```python
from build123d import *

# Parameters (mm, degrees)
F3_START = 7.62
F2_R     = 4.826
F3_DEPTH = 93.981
F4_R     = 1.1938
F5_DEPTH = 12.7


with BuildPart() as f1:
    # F0 (on Right) → F1 (revolve)
    with BuildSketch(Plane.YZ):
        with BuildLine():
            Line((-40.64, 3.175), (0, 3.175))
            Line((0, 3.175), (0, 12.7))
            Line((0, 12.7), (-6.35, 12.7))
            Line((-6.35, 12.7), (-6.35, 9.7636567324))
            ThreePointArc((-6.35, 9.7636567324), (-7.4331158517, 7.6830105399), (-9.758731164, 7.3768374756))
            Line((-9.758731164, 7.3768374756), (-24.384, 12.7))
            Line((-24.384, 12.7), (-99.4210244843, 12.7))
            ThreePointArc((-99.4210244843, 12.7), (-101.0513051228, 6.4427853895), (-101.6, 0))
            Line((-101.6, 0), (-40.64, 0))
            Line((-40.64, 0), (-40.64, 3.175))
        make_face()
    revolve(axis=Axis((0, -71.12, 0), (0, -1, 0)))

    # F2 (on Front) → F3 (cut)
    with BuildSketch(Plane.XZ.offset(F3_START)):
        with Locations((-0.1624401561, 16.0011754942)):
            Circle(F2_R)
        with Locations((13.7762043903, 8.1412650489)):
            Circle(F2_R)
        with Locations((13.9386445464, -7.8599104453)):
            Circle(F2_R)
        with Locations((0.1624401561, -16.0011754942)):
            Circle(F2_R)
        with Locations((-13.7762043903, -8.1412650489)):
            Circle(F2_R)
        with Locations((-13.9386445464, 7.8599104453)):
            Circle(F2_R)
    extrude(amount=F3_DEPTH, mode=Mode.SUBTRACT)

    # F4 (on Top) → F5 (cut, symmetric)
    with BuildSketch(Plane.XY):
        with Locations((0, -33.274)):
            Circle(F4_R)
    extrude(amount=F5_DEPTH, both=True, mode=Mode.SUBTRACT)


solid = f1.part
```
CAD build for the part. Positions are in the model's coordinates, mm. A direction names the side the tool comes from. Round coordinates to 2 decimals unless told otherwise and drop trailing zeros. Write each loop counter-clockwise with the first axis right and the second up, starting at its lowest first coordinate (ties: lowest second). Pieces come first, ordered by that corner, then holes. Notation, with made-up numbers: (70, 80.25) - (108, 80.25) arc R31 ccw to (108, 113.25) - close; hole circle Ø2 at (-16.5, 21). An arc over 180 degrees is marked (long way). Write item = value, one per line. Start each with the question number.
Q1. Which spindle directions (+Z, -Z, +X, -X, +Y, -Y) get a long thin tool onto all of the face, cutting with end or side? Do faces 5 (the cylindrical face through (0.161, -59.501, -11.175)), 6 (the conical face through (7.89, -13.92, 4.1)), 7 (the cylindrical face through (-0.161, -59.503, 11.175)), 8 (the cylindrical face through (9.758, -59.502, -5.448)). Say none if no direction does.
Q2. Probe L1, parallel to X at y = -28.5, z = 0 (3 decimals); L2, parallel to X at y = -21, z = 0.5; L3, parallel to Z at x = 0, y = -12 (3 decimals). List the from-to ranges inside material, lowest first. Write a range as from..to.
Q3. Mould opens along Z. For faces 1 (the cylindrical face through (2.8, -20, 1.5)), 2 (the cylindrical face through (-6.42, -62.43, 10.96)), 3 (the cylindrical face through (-12.7, -62.4, -0.1)), 4 (the cylindrical face through (-9.758, -59.502, 5.448)) say: pulls with the +Z half, pulls with the -Z half, needs draft (parallel to the pull), parting line crosses it, or undercut.
Q4. Band-saw the part on A-A (y = -72.5). Give the cut face in (x, z).
Q5. Band-saw the part on B-B (x = 0). Give the cut face in (y, z) (3 decimals).
Q6. Drop flat-ended pins along their axis: pin 1 (3 mm diameter, centred on x = 0, y = -33.274, fed in from -Z); pin 2 (10 mm diameter, centred on x = -5, y = -29.5, fed in from +Z); pin 3 (12 mm diameter, centred on x = 1.5, y = -43, fed in from -Z); pin 4 (12 mm diameter, centred on y = -60.5, z = -4, fed in from +X). Give the stop position or say it passes through.
Q7. Band-saw the part on C-C (z = 0). Give the cut face in (x, y) (3 decimals).
Answers below:
q1.face_5 = -Z, -Y
q1.face_6 = none
q1.face_7 = +Z, -Y
q1.face_8 = +X, -Y
q2.L1 = -12.7..-3.175, 3.175..12.7
q2.L2 = -11.46..-3.14, 3.14..11.46
q2.L3 = -8.193..-3.175, 3.175..8.193
q3.face_1 = undercut
q3.face_2 = pulls with the +Z half
q3.face_3 = parting line crosses it
q3.face_4 = undercut
q4.outline = (-12.25, 3.34) arc R12.7 ccw to (-12.18, -3.59) arc R4.83 cw to (-9.02, -8.94) arc R12.7 ccw to (-2.99, -12.34) arc R4.83 cw to (3.24, -12.28) arc R12.7 ccw to (9.2, -8.76) arc R4.83 cw to (12.25, -3.34) arc R12.7 ccw to (12.18, 3.59) arc R4.83 cw to (9.02, 8.94) arc R12.7 ccw to (2.99, 12.34) arc R4.83 cw to (-3.24, 12.28) arc R12.7 ccw to (-9.2, 8.76) arc R4.83 cw to start
q5.outline = (-99.923, -11.178) - (-34.468, -11.178) - (-34.468, -3.175) - (-40.64, -3.175) - (-40.64, 3.175) - (-34.468, 3.175) - (-34.468, 11.178) - (-99.923, 11.178) arc R38.1 ccw to start; (-32.08, -11.178) - (-20.202, -11.178) - (-9.759, -7.377) arc R2.54 cw to (-6.35, -9.764) - (-6.35, -12.7) - (0, -12.7) - (0, -3.175) - (-32.08, -3.175) - close; (-32.08, 3.175) - (0, 3.175) - (0, 12.7) - (-6.35, 12.7) - (-6.35, 9.764) arc R2.54 cw to (-9.759, 7.377) - (-20.202, 11.178) - (-32.08, 11.178) - close
q6.pin_1 = -11.47
q6.pin_2 = 12.28
q6.pin_3 = -12.34
q6.pin_4 = 12.7
q7.outline = (-12.7, -99.421) arc R38.1 ccw to (12.7, -99.421) - (12.7, -24.384) - (7.377, -9.759) arc R2.54 cw to (9.764, -6.35) - (12.7, -6.35) - (12.7, 0) - (3.175, 0) - (3.175, -40.64) - (-3.175, -40.64) - (-3.175, 0) - (-12.7, 0) - (-12.7, -6.35) - (-9.764, -6.35) arc R2.54 cw to (-7.377, -9.759) - (-12.7, -24.384) - close
